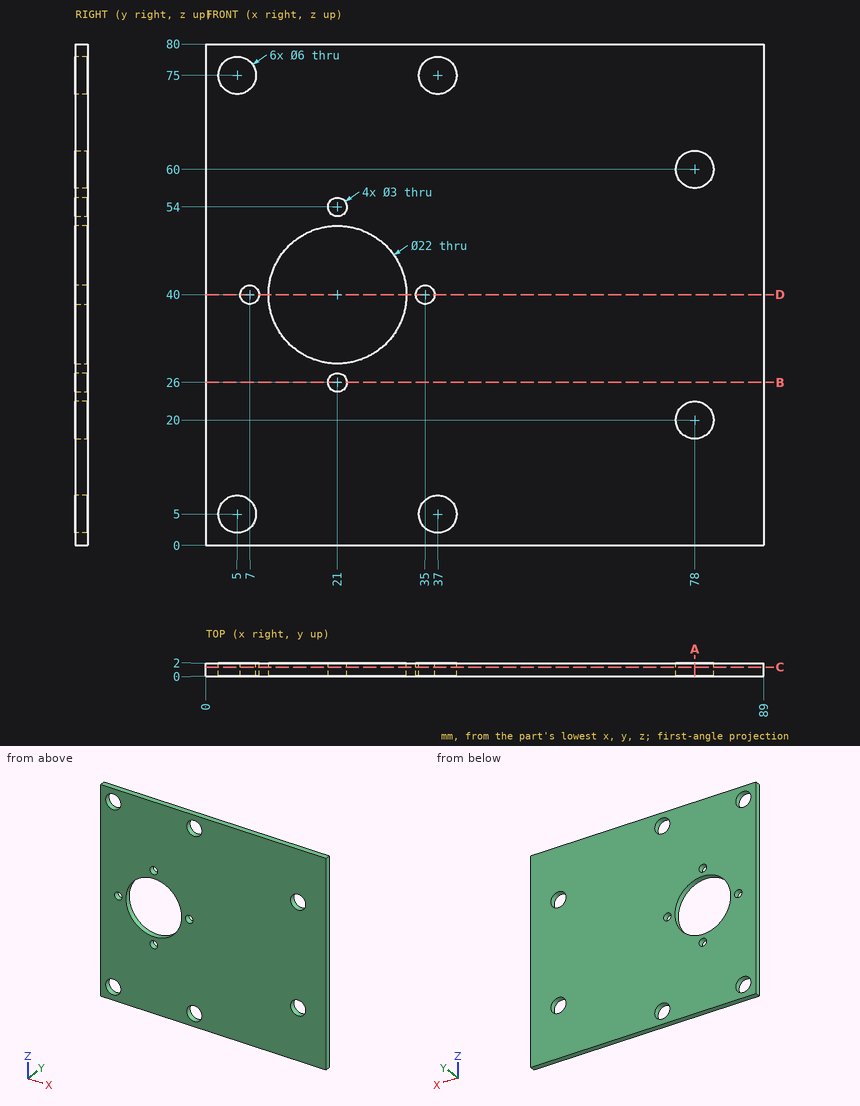
Design review of the part shown in the three views and the two pictorial views. Dimensions are in mm from the part's minimum x, y and z. Give positions to 0.01 mm unless a question says otherwise; leave off trailing zeros. Write each loop counter-clockwise with the first axis right and the second up, starting at its lowest first coordinate (ties: lowest second). Pieces come first, ordered by that corner, then holes. Notation, with made-up numbers: M -37,64 L 6,64 A30 cw 6,101 Z; hole C 36,18 d11. An arc over 180 degrees is marked long. Return JSON: item names as keys, results as strings. Group by question number.
Item 1: Wall thickness on line 1 along X through (y, z) = (0.6, 26); line 2 along X through (y, z) = (0.85, 21.5); line 3 along Z through (x, y) = (13, 0.25): over which ranges is each line inside the solid? List them lowest first.
Item 2: Take a section at A-A (x = 78). Give the boundary of the cut face in (y, z).
Item 3: Take a section at B-B (z = 26). Give the boundary of the cut face in (x, y), plus the area to 3 significant figures.
Item 4: Take a section at C-C (y = 1.4). Count the separate pieces of the cut face and the enclosed holes in it, plus the area to 3 significant figures.
Item 5: Take a section at D-D (z = 40). Give the boundary of the cut face in (x, y).
Return value:
{
 "1": {"line 1": "x = 0 to 19.5, 22.5 to 89", "line 2": "x = 0 to 75.4, 80.6 to 89", "line 3": "z = 0 to 32.45, 47.55 to 80"},
 "2": {"outline": "M 0,0 L 2,0 L 2,17 L 0,17 Z; M 0,23 L 2,23 L 2,57 L 0,57 Z; M 0,63 L 2,63 L 2,80 L 0,80 Z"},
 "3": {"outline": "M 0,0 L 19.5,0 L 19.5,2 L 0,2 Z; M 22.5,0 L 89,0 L 89,2 L 22.5,2 Z", "area": "172 mm2"},
 "4": {"separate pieces": "1", "enclosed holes": "11", "area": "6,540 mm2"},
 "5": {"outline": "M 0,0 L 5.5,0 L 5.5,2 L 0,2 Z; M 8.5,0 L 10,0 L 10,2 L 8.5,2 Z; M 32,0 L 33.5,0 L 33.5,2 L 32,2 Z; M 36.5,0 L 89,0 L 89,2 L 36.5,2 Z"}
}
